Could you check a few things on this model? Use its own coordinates, in mm. A direction names the side the tool comes from. Coordinates: 2 decimals unless noted, no trailing zeros. Loops run counter-clockwise (first coordinate to the right, second up) from the corner with the lowest first, then second, coordinate; pieces in that order, holes last. Notation, with made-up numbers: (37, -3.5) - (80, -3.5) arc R29 ccw to (80, 32.5) - close; hole circle Ø5 at (54, -9). An arc over 180 degrees is marked (long way). One line per item, written item: value. Start each with the question number.
(1) If I drill on line 1 along X through (y, z) = (0.65, 2.5); line 2 along X through (y, z) = (1.25, 9.12); line 3 along X through (y, z) = (-0.75, 2.5), over which ranges is the centre line in solid material (lowest first)? Write a range as from..to.
(2) I'm going to push flat-ended pins straight in: P1, Ø2, axis at y = 0, z = 4.5, coming from the -X side; P2, Ø0.5, axis at x = 18, y = 1, coming from the -Z side; P3, Ø1.4, axis at y = 0.5, z = -2.5, coming from the -X side. Where does each tip first touch, or does it pass through?
(3) On a 3-axis mill with a long thin cutter (end or side, diameter ignored), from which of +Z, -Z, +X, -X, +Y, -Y can I reach the whole of each face in a straight line? I mean faces 1 (the face through (14.5, 1, -4)), 2 (the face through (18, 1, 5)), 3 (the face through (9.5, 1, 9)). Say none if no direction works.
(4) If we section it at C-C on y = 1.1: Count the separate pieces of the cut face and the enclosed holes in it, then the cut area to 3 significant figures.
(5) If we section it at A-A on z = 9.12: Write out the boundary of the cut face in (x, y), then the cut area to 3 significant figures.
(6) If we section it at B-B on x = 5.38: Write out the boundary of the cut face in (y, z).
(7) If we section it at D-D on z = 4: Write out the boundary of the cut face in (x, y), then the cut area to 3 significant figures.
```python
from build123d import *

# Parameters (mm, degrees)
EXTRUDE_1_DEPTH     = 1.78
FILLET_1_R          = 2.5
SKETCH_2_R          = 0.5
CUT_EXTRUDE_2_DEPTH = 1.78
SKETCH_4_R          = 3.535533906
SKETCH_4_R_2        = 2
EXTRUDE_2_DEPTH     = 2.44


with BuildPart() as part:
    # 草图1 → 凸台-拉伸1 (new body)
    with BuildSketch(Plane(origin=(0, 0, 0), x_dir=(1, 0, 0), z_dir=(0, 1, 0))):
        Polygon((0, 0), (9.5, 0), (9.5, 9.5), (14.5, 9.5), (14.5, 0), (24, 0), (24, -5), (14.5, -5), (14.5, -14.5), (9.5, -14.5), (9.5, -5), (0, -5), align=None)
    extrude(amount=EXTRUDE_1_DEPTH)

    # 圆角1
    fillet_1_edges = [part.edges().sort_by_distance(p)[0] for p in [
        (0, 0.89, 5),
        (0, 0.89, 0),
        (9.5, 0.89, -9.5),
        (14.5, 0.89, -9.5),
        (24, 0.89, 0),
        (24, 0.89, 5),
        (9.5, 0.89, 14.5),
        (14.5, 0.89, 14.5),
    ]]
    fillet(fillet_1_edges, radius=FILLET_1_R - 0.0001)  # a hair under: the kernel refuses the full size

    # 草图2 → 切除-拉伸2 (cut)
    with BuildSketch(Plane(origin=(0, 1.78, 0), x_dir=(1, 0, 0), z_dir=(0, 1, 0))):
        with Locations(Location((2.6, -2.5, 0), (0, 0, 270))):
            Circle(SKETCH_2_R)
        with Locations(Location((5.38, -2.5, 0), (0, 0, 270))):
            Circle(SKETCH_2_R)
        with Locations(Location((12, 6.9, 0), (0, 0, 270))):
            Circle(SKETCH_2_R)
        with Locations(Location((12, 4.12, 0), (0, 0, 270))):
            Circle(SKETCH_2_R)
        with Locations(Location((21.4, -2.5, 0), (0, 0, 270))):
            Circle(SKETCH_2_R)
        with Locations(Location((18.62, -2.5, 0), (0, 0, 270))):
            Circle(SKETCH_2_R)
        with Locations(Location((12, -11.9, 0), (0, 0, 270))):
            Circle(SKETCH_2_R)
        with Locations(Location((12, -9.12, 0), (0, 0, 270))):
            Circle(SKETCH_2_R)
    extrude(amount=-CUT_EXTRUDE_2_DEPTH, mode=Mode.SUBTRACT)

    # 草图4 → 凸台-拉伸2 (add)
    with BuildSketch(Plane.XZ):
        with Locations(Location((12, 2.5, 0), (0, 0, 45))):
            Circle(SKETCH_4_R)
        with Locations(Location((12, 2.5, 0), (0, 0, 270))):
            Circle(SKETCH_4_R_2, mode=Mode.SUBTRACT)
    extrude(amount=EXTRUDE_2_DEPTH)


solid = part.part
```
Values:
1. line 1: x = 0..2.1, 3.1..4.88, 5.88..18.12, 19.12..20.9, 21.9..24
1. line 2: x = 9.5..11.5, 12.5..14.5
1. line 3: x = 8.46..10, 14..15.54
2. P1: stops at x = 0.21
2. P2: stops at z = 0
2. P3: stops at x = 9.5
3. face 1: -Z, +X, +Y, -Y
3. face 2: +Z, +X, +Y, -Y
3. face 3: +Z, -X, +Y, -Y
4. separate pieces: 1
4. enclosed holes: 8
4. area: 198 mm2
5. outline: (9.5, 0) - (11.5, 0) - (11.5, 1.78) - (9.5, 1.78) - close; (12.5, 0) - (14.5, 0) - (14.5, 1.78) - (12.5, 1.78) - close
5. area: 7.12 mm2
6. outline: (0, 0) - (1.78, 0) - (1.78, 2) - (0, 2) - close; (0, 3) - (1.78, 3) - (1.78, 5) - (0, 5) - close
7. outline: (0.5, 0) - (8.8, 0) - (8.8, -2.44) - (10.68, -2.44) - (10.68, 0) - (13.32, 0) - (13.32, -2.44) - (15.2, -2.44) - (15.2, 0) - (23.5, 0) - (23.5, 1.78) - (0.5, 1.78) - close
7. area: 50.1 mm2
